Source: CAD feature listing. Evaluate the final solid. Frame: model axes, mm. A direction names the side the tool comes from. Give positions to 0.01 mm unless a question says otherwise; leave off trailing zeros. Write each loop counter-clockwise with the first axis right and the second up, starting at its lowest first coordinate (ties: lowest second). Pieces come first, ordered by that corner, then holes. Notation, with made-up numbers: M -36.75,37 L -2.75,37 A29 ccw -2.75,61 Z; hole C 83,5 d1. An arc over 180 degrees is marked long. Return JSON: item names as keys, results as strings.
Autodesk Inventor part; units mm, degrees
ref_plane "YZ Plane" through (0, 0, 0) normal (1, 0, 0) x (0, 1, 0)
ref_plane "XZ Plane" through (0, 0, 0) normal (0, 1, 0) x (-1, 0, 0)
ref_plane "XY Plane" through (0, 0, 0) normal (0, 0, 1) x (1, 0, 0)
sketch "Sketch1" plane through (0, 0, 0) normal (0, 0, 1) x (1, 0, 0)
  line L0 (0, 0) -> (12.7, 0)
  line L1 (12.7, 0) -> (12.7, 31.75)
  line L2 (12.7, 31.75) -> (0, 31.75)
  line L3 (0, 12.7) -> (0, 0)
  line L4 (12.7, 31.75) -> (-12.7, 31.75)
  line L5 (-12.7, 31.75) -> (-12.7, 12.7)
  line L6 (-12.7, 12.7) -> (0, 12.7)
  line L7 (12.7, 12.7) -> (12.7, 31.75)
  dimension "d1" = 31.75
  dimension "d2" = 25.4
  dimension "d3" = 19.05
  dimension "d4" = 12.7
  dimension "d5" = 12.7
extrude "Extrusion1" add sketch "Sketch1" along normal blind 6.35
fillet "Fillet1" radius 19.05 1 edges at (-12.7, 31.75, 3.175)
sketch "Sketch2" plane through (0, 0, 6.35) normal (0, 0, 1) x (1, 0, 0)
  line L0 (12.7, 0) -> (12.7, 31.75)
  line L1 (0, 0) -> (12.7, 0)
  point P0 (6.35, 6.35)
  dimension "d11" = 6.35
  dimension "d12" = 6.35
hole "Hole1" at (6.35, 6.35, 6.35) direction (0, 0, -1) diameter 6.604 end through all
sketch "Sketch3" plane through (0, 0, 6.35) normal (0, 0, 1) x (1, 0, 0)
  line L0 (12.7, 0) -> (12.7, 31.75)
  line L1 (12.7, 31.75) -> (6.35, 31.75)
  point P0 (0, 0)
  point P1 (6.35, 25.4)
  dimension "d20" = 6.35
  dimension "d21" = 6.35
hole "Hole2" at (6.35, 25.4, 6.35) direction (0, 0, -1) diameter 2.159 end through all
sketch "Sketch4" plane through (0, 0, 6.35) normal (0, 0, 1) x (1, 0, 0)
  circle A0 centre (6.35, 6.35) radius 3.302
  circle A1 centre (6.35, 6.35) radius 19.05
  line L0 (-7.1204, 19.8204) -> (6.35, 6.35)
  line L1 (12.7, 0) -> (12.7, 31.75)
  point P0 (0, 0)
  dimension "d29" = 38.1
  dimension "d30" = 45
hole "Hole3" at (-7.1204, 19.8204, 6.35) direction (0, 0, -1) diameter 2.6416 end through all
properties part number "Shooter_Stop"
1) Contact query for flat-ended pins moving along their axis: pin 1 Ø2 at (x, y) = (-7.12, 19.82) entering from -Z; pin 2 Ø1.5 at (x, z) = (-8, 1.5) entering from +Y; pin 3 Ø1.9 at (y, z) = (6, 2.5) entering from -X. Output: stop coordinate, or through.
Numbers:
{"pin 1": "passes through", "pin 2": "stops at y = 26.04", "pin 3": "stops at x = 0"}
2) Cut plane A-A, the plane y = 6.35. Return the cut outline in (x, z).
Numbers:
{"outline": "M 0,0 L 3.05,0 L 3.05,6.35 L 0,6.35 Z; M 9.65,0 L 12.7,0 L 12.7,6.35 L 9.65,6.35 Z"}
3) Draft query along Y for faces 1 (the face through (9.573, 7.066, 3.131)), 2 (the face through (10, 31.75, 3)), 3 (the face through (3, 20, 6.35)). Return one class per face: released by +Y, released by -Y, zero draft, split by the parting line, or undercut.
Numbers:
{"face 1": "undercut", "face 2": "released by +Y", "face 3": "zero draft"}
4) Cut plane B-B, the plane z = 1.5. Give the number of separate pieces and of enclosed holes in the cut face, then the cut area to 3 significant figures.
Numbers:
{"separate pieces": "1", "enclosed holes": "3", "area": "524 mm²"}
5) Set-up query: faces 4 (the face through (6, 0, 3)), 5 (the face through (-6, 12.7, 3)). Return all of +Z, -Z, +X, -X, +Y, -Y with unobstructed straight access to the full face (end or side cutting, diameter ignored); none if empty.
Numbers:
{"face 4": "+Z, -Z, +X, -X, -Y", "face 5": "+Z, -Z, -X, -Y"}
6) Line query: line 1 (Y direction, x = 6.35, z = 1.75); line 2 (X direction, y = 6.35, z = 4); line 3 (X direction, y = 11, z = 2.5). Output: solid intervals per line, ascending. Write a range as [from, to].
Numbers:
{"line 1": "y = [0, 3.05], [9.65, 24.32], [26.48, 31.75]", "line 2": "x = [0, 3.05], [9.65, 12.7]", "line 3": "x = [0, 12.7]"}
